Can you work these out from the model? Positions are in its coordinate system, mm. Face numbers are marked on the shaded views. A direction names the side the tool comes from. Give positions to 0.01 mm unless a question says otherwise; leave off trailing zeros. Loops run counter-clockwise (first coordinate to the right, second up) from the corner with the lowest first, then second, coordinate; pieces in that order, holes last. Notation, with made-up numbers: (3, 36) -> (49, 36) arc R19 cw to (49, 67) -> close; hole circle Ø10 at (-28, -12). An arc over 180 degrees is marked (long way). One line per question, with ' | ' between items.
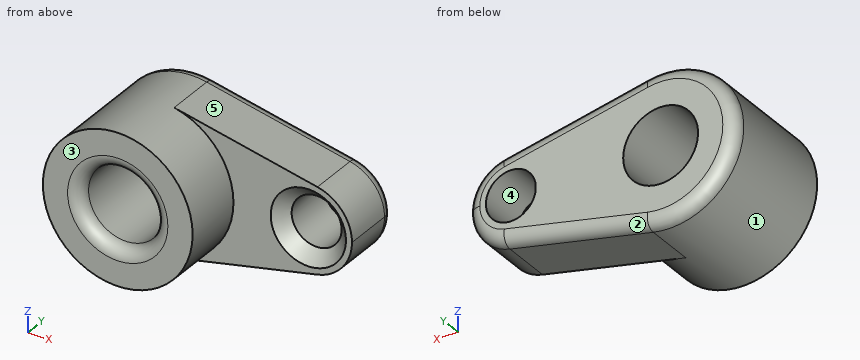
from build123d import *

# Parameters (mm, degrees)
F0_R     = 15
F0_R_2   = 10
F1_DEPTH = 25
F2_DEPTH = 50
F3_R     = 5.08
F4_SIZE  = 5.08


with BuildPart() as f1:
    # F0 (on Front) → F1 (new body)
    with BuildSketch(Plane.XZ):
        with BuildLine():
            ThreePointArc((-48.8587082131, -29.3417364858), (-31.7902605804, -18.8745860882), (-25.1087082131, 0))
            ThreePointArc((-25.1087082131, 0), (-31.7902605804, 18.8745860882), (-48.8587082131, 29.3417364858))
            ThreePointArc((-48.8587082131, 29.3417364858), (-85.1087082131, 0), (-48.8587082131, -29.3417364858))
        make_face()
        with Locations((-55.1087082131, 0)):
            Circle(F0_R, mode=Mode.SUBTRACT)
        with BuildLine():
            ThreePointArc((-48.8587082131, 29.3417364858), (-31.7902605804, 18.8745860882), (-25.1087082131, 0))
            ThreePointArc((-25.1087082131, 0), (-31.7902605804, -18.8745860882), (-48.8587082131, -29.3417364858))
            Line((-48.8587082131, -29.3417364858), (8.5371251202, -17.11601295))
            ThreePointArc((8.5371251202, -17.11601295), (-12.6087082131, 0), (8.5371251202, 17.11601295))
            Line((8.5371251202, 17.11601295), (-48.8587082131, 29.3417364858))
        make_face()
        with BuildLine():
            ThreePointArc((22.3912917869, 0), (18.4937195726, 11.0101752181), (8.5371251202, 17.11601295))
            ThreePointArc((8.5371251202, 17.11601295), (-12.6087082131, 0), (8.5371251202, -17.11601295))
            ThreePointArc((8.5371251202, -17.11601295), (18.4937195726, -11.0101752181), (22.3912917869, 0))
        make_face()
        with Locations((4.8912917869, 0)):
            Circle(F0_R_2, mode=Mode.SUBTRACT)
    extrude(amount=F1_DEPTH)

    # F0 (on Front) → F2 (join)
    with BuildSketch(Plane.XZ):
        with BuildLine():
            ThreePointArc((-48.8587082131, -29.3417364858), (-31.7902605804, -18.8745860882), (-25.1087082131, 0))
            ThreePointArc((-25.1087082131, 0), (-31.7902605804, 18.8745860882), (-48.8587082131, 29.3417364858))
            ThreePointArc((-48.8587082131, 29.3417364858), (-85.1087082131, 0), (-48.8587082131, -29.3417364858))
        make_face()
        with Locations((-55.1087082131, 0)):
            Circle(F0_R, mode=Mode.SUBTRACT)
    extrude(amount=F2_DEPTH)

    # F3
    f3_edges = [f1.edges().sort_by_distance(p)[0] for p in [
        (-70.108708, -50, 0),
        (-20.160792, 0, -23.228875),
    ]]
    fillet(f3_edges, radius=F3_R)

    # F4
    f4_edges = [f1.edges().sort_by_distance(p)[0] for p in [
        (-38.620811, -48.512102, 0),
        (-70.108708, -44.92, 0),
        (-75.188708, -50, 0),
        (-5.108708, -25, 0),
    ]]
    chamfer(f4_edges, length=F4_SIZE)


solid = f1.part
Q1. On a 3-axis mill with a long thin cutter (end or side, diameter ignored), from which of +Z, -Z, +X, -X, +Y, -Y can I reach the whole of each face in a straight line? I mean the marked faces 1 and 2. Say none if no direction works.
Entries:
face 1: -Y | face 2: -Z, +X, +Y
Q2. If we mould it in two halves opening along Z, with no side actions, what happens to the marked faces 3, 4 and 5? For each: pulls with the +Z half, pulls with the -Z half, needs draft (parallel to the pull), parting line crosses it, or undercut.
Entries:
face 3: needs draft | face 4: undercut | face 5: pulls with the +Z half
Q3. If we section it at B-B (y = -42): Write out the boundary of the cut face in (x, z).
Entries:
outline: circle Ø60 at (-55.11, 0); hole circle Ø30 at (-55.11, 0)
Q4. If we section it at A-A (y = -10.5): Write out the boundary of the cut face in (x, z), plus the area to 3 significant figures.
Entries:
outline: (-48.86, -29.34) -> (8.54, -17.12) arc R17.5 ccw to (8.54, 17.12) -> (-48.86, 29.34) arc R30 ccw (long way) to start; hole circle Ø30 at (-55.11, 0); hole circle Ø20 at (4.89, 0) | area: 3,790 mm²
Q5. For pin 1 Ø8 at (y, z) = (-27, -15) entering from -X; pin 2 Ø6 at (x, z) = (-26, -8) entering from +Y; pin 3 Ø8 at (x, z) = (-28.5, -21.5) entering from -Y; pin 4 Ø5 at (y, z) = (-18.5, 6) entering from +X, each with a flat end and sliding along its axis, tell me the tip position at first contact or that it passes through.
Entries:
pin 1: x = -83.02 | pin 2: y = 0 | pin 3: y = -25 | pin 4: x = 22.04
Q6. If we section it at C-C (y = -3.5): Write out the boundary of the cut face in (x, z).
Entries:
outline: (-48.91, -29.1) -> (8.48, -16.87) arc R17.25 ccw to (8.48, 16.87) -> (-48.91, 29.1) arc R29.75 ccw (long way) to start; hole circle Ø30 at (-55.11, 0); hole circle Ø20 at (4.89, 0)
Q7. If I drill on probe 1 along X at (y, z) = (-22, -6); probe 2 along X at (y, z) = (-7.5, 6); probe 3 along Z at (x, y) = (-66, -46.5), over which ranges is the centre line in solid material (lowest first)? Write a range as from..to.
Entries:
probe 1: -84.5..-68.86, -41.36..-5.59, 15.38..21.33 | probe 2: -84.5..-68.86, -41.36..-3.11, 12.89..21.33 | probe 3: -27.95..-10.68, 10.68..27.95
